Design review of the part built by this model. Coordinates are the model's own, in mm. A direction names the side the tool comes from. Coordinates: 2 decimals unless noted, no trailing zeros. Loops run counter-clockwise (first coordinate to the right, second up) from the corner with the lowest first, then second, coordinate; pieces in that order, holes last. Notation, with made-up numbers: M -30.5,66.5 L -15.5,66.5 A25 ccw -15.5,82.5 Z; hole C 87,13 d3. An arc over 180 degrees is marked long. Answer as CSV lines item,"result". Start each with the question number.
Autodesk Fusion 360 part; units mm, degrees
sketch "Sketch1" plane through (0, 0, 0) normal (0, 1, 0) x (1, 0, 0)
  circle A0 centre (0, 0) radius 63.5
  circle A1 centre (0, 0) radius 6.35
extrude "Extrude1" add sketch "Sketch1" along normal blind 45.72 makes body 1
sketch "Sketch2" plane through (0, 0, 0) normal (0, -1, 0) x (1, 0, 0)
  circle A0 centre (0, 0) radius 6.35
  circle A1 centre (0, 0) radius 63.5
  circle A2 centre (0, 0) radius 50.8
  circle A3 centre (0, 0) radius 19.05
  dimension "d5" = 101.6
  dimension "d6" = 38.1
extrude "Extrude2" cut sketch "Sketch2" against normal blind 3.175 contours A2 bodies 1
sketch "Sketch3" plane through (0, 45.72, 0) normal (0, 1, 0) x (-1, 0, 0)
  circle A0 centre (0, 0) radius 6.35
  circle A1 centre (0, 0) radius 63.5
  circle A2 centre (0, 0) radius 50.8
  circle A3 centre (0, 0) radius 19.05
  dimension "d9" = 101.6
  dimension "d10" = 38.1
extrude "Extrude3" cut sketch "Sketch3" against normal blind 3.175 contours A2 bodies 1
fillet "Fillet1" radius 3.175 2 edges at (17.7608, 42.545, -6.8888) (47.3622, 42.545, 18.3701) on bodies 1
fillet "Fillet2" radius 3.175 2 edges at (-17.7608, 3.175, -6.8888) (-47.3622, 3.175, 18.3701) on bodies 1
copy_body "Body->Comp1" bodies 1 removing the originals makes body 2 in component "Rolling Wheel"
component "Rolling Wheel" placed x (1, 0, 0) y (0, 1, 0) z (0, 0, 1) at (0, 0, 0)
equation "d7 = ( -1 / 4 / 2 ) * 1 in"
Item 1: Add section D-D (z = 55). Give the boundary of the cut face in (x, y), plus the area to 3 significant figures.
Item 2: For pin 1 (10 mm diameter, centred on x = -15, z = 42.5, fed in from +Y); pin 2 (6 mm diameter, centred on x = 11, z = -28, fed in from -Y) (3 decimals); pin 3 (12 mm diameter, centred on x = -16.5, y = 39, fed in from -Z), all flat-tipped, find the tip position at first contact; note any pin that passes through.
Item 3: Add section C-C (y = 30.5). Give the boundary of the cut face in (x, z).
Item 4: For line 1 along Z through (x, y) = (0.5, 32.5); line 2 along X through (y, z) = (15, 0); line 3 along Z through (x, y) = (-4, 29.5), list the stretches that pass through material, from the lowest coordinate up. Write a range as from..to.
Item 5: For faces 4 (the face through (-21, 42.545, -10)), 5 (the face through (-29, 0, -43)), list the 3-axis set-ups (+Z, -Z, +X, -X, +Y, -Y) from which the entire face can be reached by the end or side of a thin tool; tool diameter is ignored.
Item 6: Mouldability with a two-part tool opening along X and no side actions: class faces 1 (the face through (21, 3.175, -10)), 2 (the face through (-13.77, 22.54, -61.99)), 3 (the face through (-5, 0, -5)) as released by +X, released by -X, zero draft, split by the parting line, or undercut.
Response:
1,outline,"M -31.74,0 L 31.74,0 L 31.74,45.72 L -31.74,45.72 Z"
1,area,"2,900 mm²"
2,pin 1,"y = 43.69"
2,pin 2,"y = 3.175"
2,pin 3,"z = -62.63"
3,outline,"C 0,0 d127; hole C 0,0 d12.7"
4,line 1,"-63.5..-6.33, 6.33..63.5"
4,line 2,"-63.5..-6.35, 6.35..63.5"
4,line 3,"-63.37..-4.93, 4.93..63.37"
5,face 4,"+Y"
5,face 5,"+Z, -Z, +X, -X, -Y"
6,face 1,"undercut"
6,face 2,"split by the parting line"
6,face 3,"zero draft"
